CAD build for the part. Positions are in the model's coordinates, mm. Face numbers are marked on the shaded views. Coordinates: 2 decimals unless noted, no trailing zeros. Order: outer loops, then holes, each group sorted by start corner. A loop starts at its lowest first (then second) coordinate and runs counter-clockwise, first axis right, second up. Notation, with made-up numbers: (1.5, 88) - (59.5, 88) arc R16 cw to (59.5, 111) - close; hole circle Ø8 at (-1, 47.5). An arc over 180 degrees is marked (long way). Use one line per item in the form item = value.
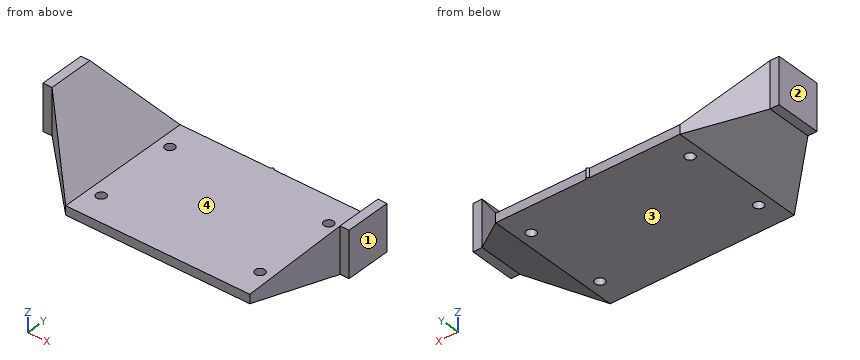
```python
from build123d import *

# Parameters (mm, degrees)
F0_R       = 1.6
F1_DEPTH   = 3
F3_W       = 15.25
F3_H       = 15.25
F4_DEPTH   = 3
F4_FACE_W  = 15.25
F4_FACE_H  = 15.25
F1_FACE_W  = 46
F1_FACE_H  = 3
F7_W       = 15.25
F7_H       = 15.25
F8_DEPTH   = 3
F8_FACE_W  = 15.25
F8_FACE_H  = 15.25
F1_FACE1_W = 46
F1_FACE1_H = 3


with BuildPart() as f1:
    # F0 (on Top) → F1 (new body)
    with BuildSketch(Plane.XY):
        with BuildLine():
            ThreePointArc((-0.5, 23), (0, 22.5), (0.5, 23))
            Line((0.5, 23), (-0.5, 23))
        make_face()
        with BuildLine():
            Line((-0.5, 23), (0.5, 23))
            ThreePointArc((0.5, 23), (0, 23.5), (-0.5, 23))
        make_face()
        with BuildLine():
            Line((30.5, 23), (0.5, 23))
            ThreePointArc((0.5, 23), (0, 22.5), (-0.5, 23))
            Line((-0.5, 23), (-30.5, 23))
            Line((-30.5, 23), (-30.5, -23))
            Line((-30.5, -23), (30.5, -23))
            Line((30.5, -23), (30.5, 23))
        make_face()
        with Locations((-26.3, -13.8)):
            Circle(F0_R, mode=Mode.SUBTRACT)
        with Locations((26.3, -13.8)):
            Circle(F0_R, mode=Mode.SUBTRACT)
        with Locations((-26.3, 13.8)):
            Circle(F0_R, mode=Mode.SUBTRACT)
        with Locations((26.3, 13.8)):
            Circle(F0_R, mode=Mode.SUBTRACT)
    extrude(amount=F1_DEPTH)



with BuildPart() as f4:
    # F3 (on offset) → F4 (new body)
    with BuildSketch(Plane.YZ.offset(47.7)):
        with Locations((0, 16.225)):
            Rectangle(F3_W, F3_H)
    extrude(amount=F4_DEPTH)


with BuildPart() as f1_1:
    add(f1.part)

    add(f4.part)  # F5 merges F4
    # F4_face (on face) → F5 section 0
    with BuildSketch(Plane(origin=(47.7, 0, 16.225), x_dir=(0, 1, 0), z_dir=(-1, 0, 0))):
        Rectangle(F4_FACE_W, F4_FACE_H)
    # F1_face (on face) → F5 section 1
    with BuildSketch(Plane(origin=(30.5, 0, 1.5), x_dir=(0, 1, 0), z_dir=(1, 0, 0))):
        Rectangle(F1_FACE_W, F1_FACE_H)
    loft()



with BuildPart() as f8:
    # F7 (on offset) → F8 (new body)
    with BuildSketch(Plane(origin=(-47.7, 0, 0), x_dir=(0, -1, 0), z_dir=(-1, 0, 0))):
        with Locations((0, 16.225)):
            Rectangle(F7_W, F7_H)
    extrude(amount=F8_DEPTH)


with BuildPart() as f1_2:
    add(f1_1.part)

    add(f8.part)  # F9 merges F8
    # F8_face (on face) → F9 section 0
    with BuildSketch(Plane(origin=(-47.7, 0, 16.225), x_dir=(0, -1, 0), z_dir=(1, 0, 0))):
        Rectangle(F8_FACE_W, F8_FACE_H)
    # F1_face1 (on face) → F9 section 1
    with BuildSketch(Plane(origin=(-30.5, 0, 1.5), x_dir=(0, -1, 0), z_dir=(-1, 0, 0))):
        Rectangle(F1_FACE1_W, F1_FACE1_H)
    loft()


solid = f1_2.part
```
Item 1: Cut at B-B, the plane y = 13.8. State how many separate pieces and enclosed holes the cut face has, plus the area to 3 significant figures.
Derived:
separate_pieces = 3
enclosed_holes = 0
area = 301 mm²
Item 2: Drop flat-ended pins along their axis: pin 1 (3.5 mm diameter, centred on x = 49, z = 15.5, fed in from +Y); pin 2 (1.5 mm diameter, centred on x = 49, y = -0.5, fed in from -Z); pin 3 (2.5 mm diameter, centred on x = -26.3, y = 13.8, fed in from +Z); pin 4 (4 mm diameter, centred on x = -26.3, y = -13.8, fed in from +Z). Give the stop position or say it passes through.
Derived:
pin_1 = 8.03
pin_2 = 8.6
pin_3 = through
pin_4 = 3
Item 3: Two-plate mould, pull along X, no slides. Class the marked faces 1, 2, 3 and 4: +X half, -X half, draft (parallel to the pull), parting line (faces both ways), or undercut.
Derived:
face_1 = +X half
face_2 = -X half
face_3 = draft
face_4 = undercut
Item 4: Drill centre lines: line 1 (X direction, y = -19.5, z = 3.25); line 2 (X direction, y = 1.5, z = 7.25); line 3 (Z direction, x = -7, y = -1.5). Where is each one in solid material? Low to high. Write a range as [from, to].
Derived:
line_1 = [-34.42, -30.71], [30.71, 34.42]
line_2 = [-45, -34.01], [34.01, 45]
line_3 = [0, 3]
Item 5: Cut at A-A, the plane x = -26.3. Write the cut outline in (y, z).
Derived:
outline = (-23, 0) - (-15.4, 0) - (-15.4, 3) - (-23, 3) - close; (-12.2, 0) - (12.2, 0) - (12.2, 3) - (-12.2, 3) - close; (15.4, 0) - (23, 0) - (23, 3) - (15.4, 3) - close
